Part model, mm, in its own coordinate system. A direction names the side the tool comes from. Round coordinates to 2 decimals unless told otherwise and drop trailing zeros. Loops run counter-clockwise (first coordinate to the right, second up) from the corner with the lowest first, then second, coordinate; pieces in that order, holes last.
from build123d import *

# Parameters (mm, degrees)
SKETCH1_W           = 8.3
SKETCH1_H           = 8.3
BOSS_EXTRUDE1_DEPTH = 5
SKETCH2_R           = 8
BOSS_EXTRUDE2_DEPTH = 30


with BuildPart() as part:
    # Sketch1 → Boss-Extrude1 (new body)
    with BuildSketch(Plane.XY):
        with BuildLine():
            Line((0, 8), (25, 8))
            ThreePointArc((25, 8), (33, 0), (25, -8))
            Line((25, -8), (0, -8))
            ThreePointArc((0, -8), (-8, 0), (0, 8))
        make_face()
        Rectangle(SKETCH1_W, SKETCH1_H, mode=Mode.SUBTRACT)
    extrude(amount=BOSS_EXTRUDE1_DEPTH)

    # Sketch2 → Boss-Extrude2 (add)
    with BuildSketch(Plane.XY.offset(5)):
        with Locations(Location((25, 0, 0), (0, 0, 90))):
            Circle(SKETCH2_R)
    extrude(amount=BOSS_EXTRUDE2_DEPTH)


solid = part.part
1) Slice it at B-B, the plane x = 20. Give the cut face in (y, z) (3 decimals).
Values:
outline: (-8, 0) - (8, 0) - (8, 5) - (6.245, 5) - (6.245, 35) - (-6.245, 35) - (-6.245, 5) - (-8, 5) - close
2) Mould opens along X. For faces 1 (the face through (0, 4.15, 2)), 2 (the face through (4.15, 0, 2)), 3 (the face through (13, 0, 0)), 4 (the face through (-8, 0, 2)) say: released by +X, released by -X, zero draft, split by the parting line, or undercut.
Values:
face 1: undercut
face 2: undercut
face 3: zero draft
face 4: released by -X
3) Tool access for faces 5 (the face through (-4.15, 0, 2)), 6 (the face through (12, 8, 2)), 7 (the face through (32.81, -1.73, 17.26)): list every direction of +Z, -Z, +X, -X, +Y, -Y with a clear straight run to the whole face (end or side of a thin tool).
Values:
face 5: +Z, -Z
face 6: +Z, -Z, +X, -X, +Y
face 7: +Z
4) Wall check: line 1 along Z through (x, y) = (-1.5, 7.75); line 2 along X through (y, z) = (-0.75, 11); line 3 along X through (y, z) = (-3.25, 17). Give the ranges that are in metal, low to high.
Values:
line 1: z = 0 to 5
line 2: x = 17.04 to 32.96
line 3: x = 17.69 to 32.31
5) Slice it at D-D, the plane z = 13. Give the cut face in (x, y), then the cut area to 3 significant figures.
Values:
outline: circle Ø16 at (25, 0)
area: 201 mm2
6) Slice it at C-C, the plane y = 2. Give the cut face in (x, z).
Values:
outline: (-7.75, 0) - (-4.15, 0) - (-4.15, 5) - (-7.75, 5) - close; (4.15, 0) - (32.75, 0) - (32.75, 35) - (17.25, 35) - (17.25, 5) - (4.15, 5) - close
7) Slice it at A-A, the plane y = 0. Give the cut face in (x, z).
Values:
outline: (-8, 0) - (-4.15, 0) - (-4.15, 5) - (-8, 5) - close; (4.15, 0) - (33, 0) - (33, 35) - (17, 35) - (17, 5) - (4.15, 5) - close
8) Drop flat-ended pins along their axis: pin 1 Ø1.5 at (y, z) = (-1, 3) entering from +X; pin 2 Ø5 at (x, y) = (3, -0.5) entering from +Z; pin 3 Ø1.5 at (y, z) = (2.5, 14.5) entering from -X. Give the stop position or say it passes through.
Values:
pin 1: stops at x = 33
pin 2: stops at z = 5
pin 3: stops at x = 17.19
